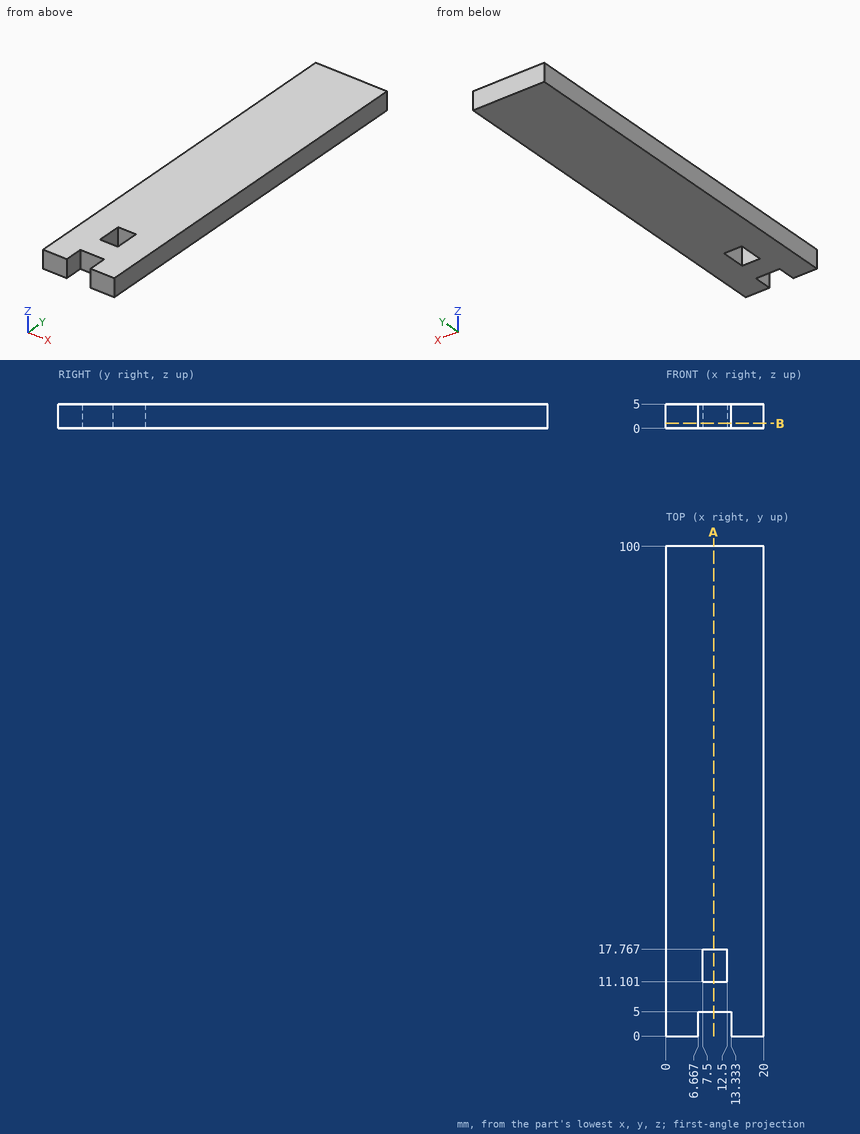
Design review of the part shown in the three views and the two pictorial views. Dimensions are in mm from the part's minimum x, y and z. Round coordinates to 2 decimals unless told otherwise and drop trailing zeros. Loops run counter-clockwise (first coordinate to the right, second up) from the corner with the lowest first, then second, coordinate; pieces in that order, holes last.
(1) We need section B-B (z = 1.05). Give the boundary of the cut face in (x, y), plus the area to 3 significant figures.
Returned:
outline: (0, 0) - (6.67, 0) - (6.67, 5) - (13.33, 5) - (13.33, 0) - (20, 0) - (20, 100) - (0, 100) - close; hole (7.5, 11.1) - (12.5, 11.1) - (12.5, 17.77) - (7.5, 17.77) - close
area: 1,930 mm2
(2) Wall thickness on line 1 along Y through (x, z) = (7.75, 1.6); line 2 along X through (y, z) = (17, 0.9); line 3 along Y through (x, z) = (6.75, 4.6): over which ranges is each line inside the solid? List them lowest first.
Returned:
line 1: y = 5 to 11.1, 17.77 to 100
line 2: x = 0 to 7.5, 12.5 to 20
line 3: y = 5 to 100
(3) We need section A-A (x = 9.75). Give the boundary of the cut face in (y, z), plus the area to 3 significant figures.
Returned:
outline: (5, 0) - (11.1, 0) - (11.1, 5) - (5, 5) - close; (17.77, 0) - (100, 0) - (100, 5) - (17.77, 5) - close
area: 442 mm2
(4) Clearance check with flat-ended pins moving along their axes: P1, Ø1.5, axis at x = 10.5, z = 3, coming from the -Y side; P2, Ø6, axis at x = 3.5, y = 55, coming from the -Z side. State where each tip first meets the part, or that it passes through.
Returned:
P1: stops at y = 5
P2: stops at z = 0
